```python
from build123d import *

# Parameters (mm, degrees)
F0_W     = 40
F0_H     = 238
F1_DEPTH = 40
F2_R     = 5
F3_W     = 30
F3_H     = 35
F4_DEPTH = 238.001
F5_W     = 20
F5_H     = 30
F6_DEPTH = 40.001
F7_W     = 30
F7_H     = 20
F8_DEPTH = 40.001


with BuildPart() as f1:
    # F0 (on Top) → F1 (new body)
    with BuildSketch(Plane.XY):
        with Locations((2.510834, 0)):
            Rectangle(F0_W, F0_H)
    extrude(amount=F1_DEPTH)

    # F2
    f2_edges = [f1.edges().sort_by_distance(p)[0] for p in [
        (22.510834, -119, 20),
        (-17.489166, -119, 20),
        (22.510834, 119, 20),
        (-17.489166, 119, 20),
    ]]
    fillet(f2_edges, radius=F2_R)

    # F3 (on face) → F4 (cut, through all)
    with BuildSketch(Plane.XZ.offset(119)):
        with Locations((2.510834, 17.5)):
            Rectangle(F3_W, F3_H)
    extrude(amount=-F4_DEPTH, mode=Mode.SUBTRACT)

    # F5 (on face) → F6 (cut, through all)
    with BuildSketch(Plane.YZ.offset(22.510834)):
        with Locations((-101.5, 20)):
            Rectangle(F5_W, F5_H)
        with Locations((-76.5, 20)):
            Rectangle(F5_W, F5_H)
        with Locations((-51.5, 20)):
            Rectangle(F5_W, F5_H)
        with Locations((-26.5, 20)):
            Rectangle(F5_W, F5_H)
        with Locations((-1.5, 20)):
            Rectangle(F5_W, F5_H)
        with Locations((23.5, 20)):
            Rectangle(F5_W, F5_H)
        with Locations((48.5, 20)):
            Rectangle(F5_W, F5_H)
        with Locations((73.5, 20)):
            Rectangle(F5_W, F5_H)
        with Locations((98.5, 20)):
            Rectangle(F5_W, F5_H)
    extrude(amount=-F6_DEPTH, mode=Mode.SUBTRACT)

    # F7 (on face) → F8 (cut, through all)
    with BuildSketch(Plane.XY.offset(40)):
        with Locations((2.510834, -101.5)):
            Rectangle(F7_W, F7_H)
        with Locations((2.510834, -76.5)):
            Rectangle(F7_W, F7_H)
        with Locations((2.510834, -51.5)):
            Rectangle(F7_W, F7_H)
        with Locations((2.510834, -26.5)):
            Rectangle(F7_W, F7_H)
        with Locations((2.510834, -1.5)):
            Rectangle(F7_W, F7_H)
        with Locations((2.510834, 23.5)):
            Rectangle(F7_W, F7_H)
        with Locations((2.510834, 48.5)):
            Rectangle(F7_W, F7_H)
        with Locations((2.510834, 73.5)):
            Rectangle(F7_W, F7_H)
        with Locations((2.510834, 98.5)):
            Rectangle(F7_W, F7_H)
    extrude(amount=-F8_DEPTH, mode=Mode.SUBTRACT)


solid = f1.part
```
Geometry: final body of the model. Coordinates: model frame, mm. A direction names the side the tool comes from. Round coordinates to 2 decimals unless told otherwise and drop trailing zeros. Loops run counter-clockwise (first coordinate to the right, second up) from the corner with the lowest first, then second, coordinate; pieces in that order, holes last. Notation, with made-up numbers: (50.5, -35) -> (56.5, -35) arc R16 cw to (56.5, -6) -> close; hole circle Ø10 at (-26.5, -32). An arc over 180 degrees is marked (long way). Use one line per item in the form item = value. Start each with the question number.
1) Draft query along Z for faces 1 (the flat face through (3, 61, 35)), 2 (the flat face through (2, 38.5, 38)), 3 (the flat face through (-15, 38.5, 20)). Return one class per face: released by +Z, released by -Z, zero draft, split by the parting line, or undercut.
2) Section A-A on y = 69.5. Output: boundary loops of the cut face in (x, z), then the cut area to 3 significant figures.
3) Access query for faces 4 (the flat face through (20, -36.5, 20)), 5 (the flat face through (17.511, -27, 38)). Directions: +Z, -Z, +X, -X, +Y, -Y. A direction counts if a zero-diameter tool reaches every point of the face in a straight line with its end or side. Return the directions, or none.
4) First-contact query: P1, Ø2.5, axis at x = -14, z = 19.5, coming from the -Y side; P2, Ø2.5, axis at x = -16, z = 17.5, coming from the +Y side; P3, Ø1.5, axis at x = -15.5, z = 19, coming from the -Y side. Flat tips, straight axial feed; report the tip coordinate or a pass-through.
5) Line query: L1, parallel to Z at x = -13.5, y = 105; L2, parallel to X at y = -47.5, z = 35.5; L3, parallel to Z at x = -1.5, y = -65.5. Output: solid intervals per line, ascending.
6) Section B-B on z = 15. Give the number of separate pieces and of enclosed holes in the cut face, then the cut area to 3 significant figures.
Response:
q1.face_1 = released by -Z
q1.face_2 = zero draft
q1.face_3 = undercut
q2.outline = (-17.49, 0) -> (-12.49, 0) -> (-12.49, 5) -> (-17.49, 5) -> close; (-17.49, 35) -> (-12.49, 35) -> (-12.49, 40) -> (-17.49, 40) -> close; (17.51, 0) -> (22.51, 0) -> (22.51, 5) -> (17.51, 5) -> close; (17.51, 35) -> (22.51, 35) -> (22.51, 40) -> (17.51, 40) -> close
q2.area = 100 mm^2
q3.face_4 = +X, -X
q3.face_5 = +Z, -Z
q4.P1 = -118.99
q4.P2 = 118.46
q4.P3 = -118.46
q5.L1 = 0 to 5, 35 to 40
q5.L2 = -17.49 to -12.49, 17.51 to 22.51
q5.L3 = 35 to 40
q6.separate_pieces = 20
q6.enclosed_holes = 0
q6.area = 559 mm^2
